Here's how the part is built. I have some questions about the finished solid (model axes, mm). A direction names the side the tool comes from. Give positions to 0.01 mm unless a question says otherwise; leave off trailing zeros. Order: outer loops, then holes, each group sorted by start corner. A loop starts at its lowest first (then second) coordinate and runs counter-clockwise, first axis right, second up. Notation, with made-up numbers: M 40,0.25 L 88,0.25 A30 ccw 88,34.25 Z; hole C 81,85.25 d10. An arc over 180 degrees is marked long. One line per item, written item: value. Start each with the question number.
from build123d import *

# Parameters (mm, degrees)
F0_W     = 19.05
F0_H     = 30.1625
F0_R     = 11.1125
F0_H_2   = 26.9875
F1_DEPTH = 12.7
F2_W     = 19.05
F2_H     = 26.9875
F3_DEPTH = 6.35
F2_H_2   = 30.1625
F4_DEPTH = 12.7


with BuildPart() as f1:
    # F0 (on Top) → F1 (new body)
    with BuildSketch(Plane.XY):
        with Locations((-47.625, 3.96875)):
            Rectangle(F0_W, F0_H)
        Polygon((0, 19.05), (-38.1, 19.05), (-38.1, -11.1125), (-38.1, -38.1), (41.275, -38.1), (41.275, 0), (57.15, 0), (57.15, 19.05), align=None)
        with Locations((0, -9.525)):
            Circle(F0_R, mode=Mode.SUBTRACT)
        with Locations((-47.625, -24.60625)):
            Rectangle(F0_W, F0_H_2)
    extrude(amount=F1_DEPTH)

    # F2 (on face) → F3 (join)
    with BuildSketch(Plane.XY.offset(12.7)):
        with Locations((-47.625, -24.60625)):
            Rectangle(F2_W, F2_H)
    extrude(amount=F3_DEPTH)

    # F2 (on face) → F4 (join)
    with BuildSketch(Plane.XY.offset(12.7)):
        with Locations((-47.625, 3.96875)):
            Rectangle(F2_W, F2_H_2)
    extrude(amount=F4_DEPTH)


solid = f1.part
Item 1: I want a section at C-C on y = 12.5. Write out the boundary of the cut face in (x, z).
Item 2: For faces 1 (the face through (-48, -11.112, 22)), 2 (the face through (-14, -9, 0)), 3 (the face through (-9, -38.1, 7)), 4 (the face through (9, 4, 12.7)), 5 (the face through (49, 0, 6)), which set-ups out of +Z, -Z, +X, -X, +Y, -Y let a thin tool reach every point of the face, with its end or its side?
Item 3: Please list where these lines run through material, in increasing order: probe 1 along Z at (x, y) = (17.5, -14); probe 2 along X at (y, z) = (-8.5, 13.5); probe 3 along Y at (x, z) = (0, 8). Write a range as [from, to].
Item 4: I want a section at A-A on x = 0. Write out the boundary of the cut face in (y, z), plus the area to 3 significant figures.
Item 5: I want a section at D-D on x = -37. Write out the boundary of the cut face in (y, z).
Item 6: Will these pins go through, and if not, where does the flat tip stop? P1, Ø10, axis at y = -15.5, z = 3.5, coming from the +X side (3 decimals); P2, Ø6.5, axis at y = -19.5, z = 19, coming from the +X side; P3, Ø8, axis at x = 43.5, y = -6, coming from the +Z side.
Item 7: We'd pull the mould along X, two halves only. Please class faces 6 (the face through (-48, 4, 25.4)), 7 (the face through (5.97, -0.15, 6.26)), 8 (the face through (-38.1, -4, 18)): +X half, -X half, draft (parallel to the pull), parting line (faces both ways), or undercut.
Answer below:
1. outline: M -57.15,0 L 57.15,0 L 57.15,12.7 L -38.1,12.7 L -38.1,25.4 L -57.15,25.4 Z
2. face 1: +Z, +X, -X, -Y
2. face 2: -Z, +X, -X, +Y, -Y
2. face 3: +Z, -Z, +X, -X, -Y
2. face 4: +Z, +X, +Y, -Y
2. face 5: +Z, -Z, +X, -Y
3. probe 1: z = [0, 12.7]
3. probe 2: x = [-57.15, -38.1]
3. probe 3: y = [-38.1, -20.64], [1.59, 19.05]
4. outline: M -38.1,0 L -20.64,0 L -20.64,12.7 L -38.1,12.7 Z; M 1.59,0 L 19.05,0 L 19.05,12.7 L 1.59,12.7 Z
4. area: 444 mm²
5. outline: M -38.1,0 L 19.05,0 L 19.05,12.7 L -38.1,12.7 Z
6. P1: stops at x = 41.275
6. P2: stops at x = -38.1
6. P3: stops at z = 12.7
7. face 6: draft
7. face 7: undercut
7. face 8: +X half
